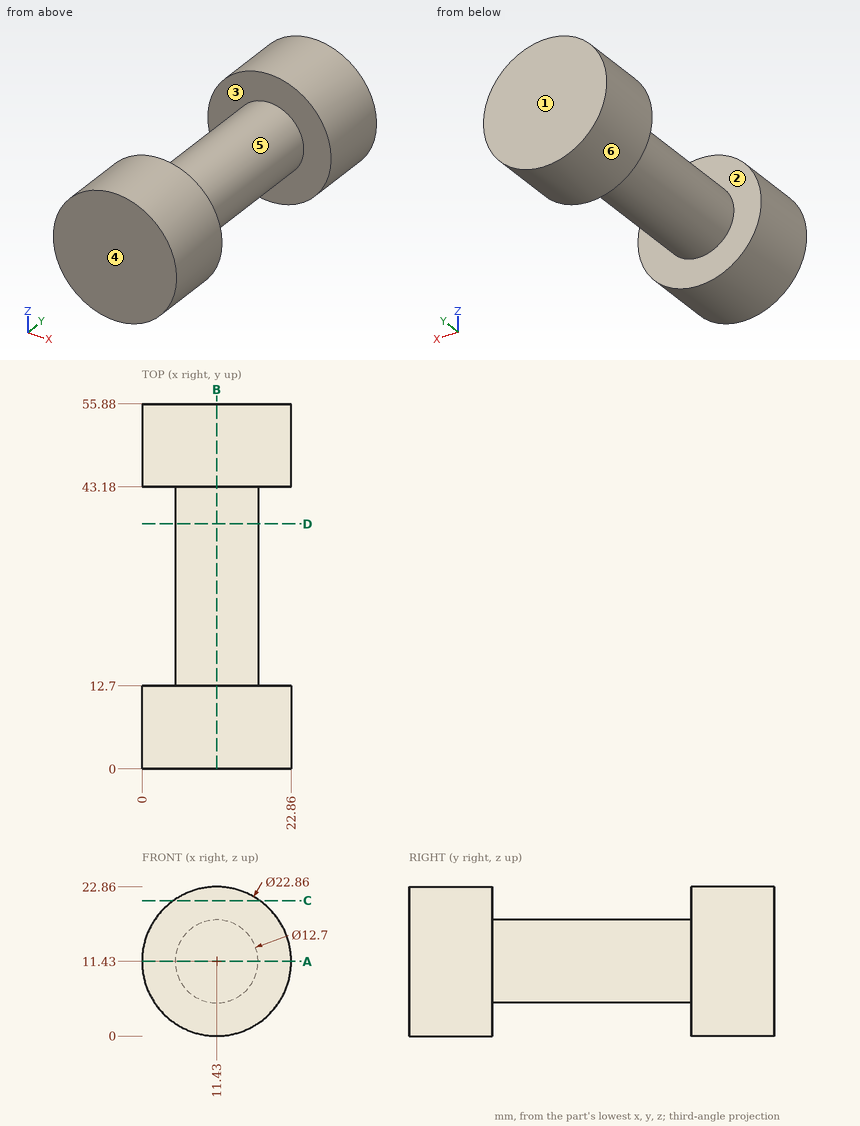
Design review of the part shown in the three views and the two pictorial views. Dimensions are in mm from the part's minimum x, y and z. A direction names the side the tool comes from. Give positions to 0.01 mm unless a question says otherwise; leave off trailing zeros. Write each loop counter-clockwise with the first axis right and the second up, starting at its lowest first coordinate (ties: lowest second). Pieces come first, ordered by that corner, then holes. Notation, with made-up numbers: M 50.5,-22.5 L 108.5,-22.5 A32 cw 108.5,9.5 Z; hole C 12,-21.75 d5. An arc over 180 degrees is marked long. One line per item, written item: value.
1) For the marked faces 1 and 2, list the 3-axis set-ups (+Z, -Z, +X, -X, +Y, -Y) from which the entire face can be reached by the end or side of a thin tool; tool diameter is ignored.
Results are:
face 1: +Z, -Z, +X, -X, +Y
face 2: none
2) Take a section at C-C, the plane z = 20.75. Write out the cut boundary in (x, y), then the cut area to 3 significant figures.
Results are:
outline: M 4.81,0 L 18.05,0 L 18.05,12.7 L 4.81,12.7 Z; M 4.81,43.18 L 18.05,43.18 L 18.05,55.88 L 4.81,55.88 Z
area: 336 mm²
3) Take a section at D-D, the plane y = 37.5. Write out the cut boundary in (x, z).
Results are:
outline: C 11.43,11.43 d12.7
4) Take a section at B-B, the plane x = 11.43. Write out the cut boundary in (y, z), then the cut area to 3 significant figures.
Results are:
outline: M 0,0 L 12.7,0 L 12.7,5.08 L 43.18,5.08 L 43.18,0 L 55.88,0 L 55.88,22.86 L 43.18,22.86 L 43.18,17.78 L 12.7,17.78 L 12.7,22.86 L 0,22.86 Z
area: 968 mm²
5) Take a section at A-A, the plane z = 11.43. Write out the cut boundary in (x, y).
Results are:
outline: M 0,0 L 22.86,0 L 22.86,12.7 L 17.78,12.7 L 17.78,43.18 L 22.86,43.18 L 22.86,55.88 L 0,55.88 L 0,43.18 L 5.08,43.18 L 5.08,12.7 L 0,12.7 Z
6) For P1, Ø5, axis at y = 38, z = 15, coming from the +X side; P2, Ø10, axis at y = 24.5, z = 19, coming from the +X side; P3, Ø1, axis at y = 45, z = 13.5, coming from the +X side, all flat-tipped, find the tip position at first contact; note any pin that passes through.
Results are:
P1: stops at x = 17.69
P2: stops at x = 17.24
P3: stops at x = 22.75
7) The part is to be moulded in two halves that separate along Y. For the marked faces 3, 4, 5 and 6, say which applies: +Y half, -Y half, draft (parallel to the pull), parting line (faces both ways), or undercut.
Results are:
face 3: undercut
face 4: -Y half
face 5: undercut
face 6: draft
8) For line 1 (Y direction, x = 11.75, z = 3.75); line 2 (X direction, y = 52.5, z = 21.5); line 3 (X direction, y = 53.5, z = 17), list the stretches that pass through material, from the lowest coordinate up. Write a range as from..to.
Results are:
line 1: y = 0..12.7, 43.18..55.88
line 2: x = 6.02..16.84
line 3: x = 1.45..21.41
